CAD build for the part. Positions are in the model's coordinates, mm. A direction names the side the tool comes from. Round coordinates to 2 decimals unless told otherwise and drop trailing zeros. Write each loop counter-clockwise with the first axis right and the second up, starting at its lowest first coordinate (ties: lowest second). Pieces come first, ordered by that corner, then holes. Notation, with made-up numbers: (-38.75, 22.25) - (16.25, 22.25) arc R16 ccw to (16.25, 50.25) - close; hole circle Ø1 at (-24, -31.75). An arc over 180 degrees is marked (long way). Use one line per item in the form item = value. Start each with the question number.
Item 1: Band-saw the part on A-A, the plane y = 50.5. List the corners of the cut face in (x, z).
Item 2: Band-saw the part on B-B, the plane x = 15. Give the number of separate pieces and of enclosed holes in the cut face, and give its area (3 significant figures).
Item 3: Tool access for faces 1 (the flat face through (26.4, 49.1, 6.6)), 2 (the flat face through (15, 65, 0.5)), 3 (the cylindrical face through (23.314, 9.721, 3.254)), 4 (the flat face through (17, 43, 5.7)): list every direction of +Z, -Z, +X, -X, +Y, -Y with a clear straight run to the whole face (end or side of a thin tool).
Item 4: Drill centre lines: L1, parallel to Y at x = 15, z = 3.05 (3 decimals); L2, parallel to Y at x = 25, z = 3; L3, parallel to Y at x = 15, z = 8.35 (3 decimals). Where is each one in solid material? Low to high.
Item 5: Pin check, flat tips, straight feed: pin 1 (3 mm diameter, centred on x = 17, y = 13.5, fed in from -Z); pin 2 (4 mm diameter, centred on x = 5, y = 65.5, fed in from +Z). Stop position of each tip, or through.
Item 6: Pull direction Y, two halves, no side cores. Call faces 5 (the flat face through (15, 0, 5)), 6 (the flat face through (12, 38, 10)), 7 (the flat face through (17, 16, 5.7)): +Y half, -Y half, draft (parallel to the pull), parting line (faces both ways), or undercut.
Autodesk Inventor part; units mm, degrees
ref_plane "YZ Plane" through (0, 0, 0) normal (1, 0, 0) x (0, 1, 0)
ref_plane "XZ Plane" through (0, 0, 0) normal (0, 1, 0) x (-1, 0, 0)
ref_plane "XY Plane" through (0, 0, 0) normal (0, 0, 1) x (1, 0, 0)
sketch "Skizze1" plane through (0, 0, 0) normal (0, 0, 1) x (1, 0, 0)
  line L0 (0, 0) -> (30, 0)
  line L1 (30, 0) -> (30, 75)
  line L2 (30, 75) -> (0, 75)
  line L3 (0, 75) -> (0, 0)
  dimension "d0" = 30
  dimension "d1" = 75
extrude "Extrusion1" add sketch "Skizze1" along normal blind 10
sketch "Skizze2" plane through (0, 0, 10) normal (0, 0, 1) x (1, 0, 0)
  line L0 (5, 65.5) -> (25, 65.5) construction
  line L1 (25, 65.5) -> (25, 50.5) construction
  line L2 (25, 50.5) -> (5, 50.5) construction
  line L3 (5, 50.5) -> (5, 65.5) construction
  line L4 (5, 9.5) -> (25, 9.5) construction
  line L5 (25, 9.5) -> (25, 24.5) construction
  line L6 (25, 24.5) -> (5, 24.5) construction
  line L7 (5, 24.5) -> (5, 9.5) construction
  line L8 (30, 75) -> (0, 75) construction
  line L9 (0, 0) -> (30, 0) construction
  line L10 (15, 65.5) -> (15, 75) construction
  line L11 (15, 50.5) -> (15, 24.5) construction
  dimension "d4" = 9.5
  dimension "d5" = 15
  dimension "d6" = 9.5
  dimension "d7" = 15
  dimension "d8" = 20
hole "Bohrung1" at (5, 65.5, 10) at (25, 65.5, 10) at (25, 50.5, 10) at (5, 50.5, 10) at (5, 24.5, 10) at (25, 24.5, 10) at (25, 9.5, 10) at (5, 9.5, 10) direction (0, 0, -1) diameter 3.4 end through all counterbore diameter 6.5 counterbore depth 3.4
sketch "Skizze4" plane through (0, 0, 0) normal (0, 0, -1) x (-1, 0, 0)
  line L0 (-18.5, 75) -> (-11.5, 75)
  line L1 (-11.5, 75) -> (-11.5, 55)
  line L2 (-11.5, 55) -> (-18.5, 55)
  line L3 (-18.5, 55) -> (-18.5, 75)
  line L4 (-30, 75) -> (0, 75)
  point P0 (0, 0)
  point P1 (-15, 75)
  dimension "d22" = 20
  dimension "d23" = 7
extrude "Extrusion3" cut sketch "Skizze4" against normal blind 0.5
fillet "Rundung1" radius 5 4 edges at (0, 75, 5) (30, 75, 5) (0, 0, 5) (30, 0, 5)
fillet "Rundung3" radius 0.5 4 edges at (18.5, 75, 0.25) (11.5, 75, 0.25) (18.5, 55, 0.25) (11.5, 55, 0.25)
fillet "Rundung2" radius 0.5 24 edges at (1.4645, 73.5355, 10) (0, 37.5, 10) (1.4645, 1.4645, 10) (15, 0, 10) (28.5355, 1.4645, 10) (30, 37.5, 10) (28.5355, 73.5355, 10) (15, 75, 10) (18.6464, 74.8536, 0) (18.5, 65, 0) (18.3536, 55.1464, 0) (15, 55, 0) (11.6464, 55.1464, 0) (11.5, 65, 0) (11.3536, 74.8536, 0) (8, 75, 0) (1.4645, 73.5355, 0) (0, 37.5, 0) (1.4645, 1.4645, 0) (15, 0, 0) (28.5355, 1.4645, 0) (30, 37.5, 0) (28.5355, 73.5355, 0) (22, 75, 0)
sketch "Skizze5" plane through (0, 0, 0) normal (0, 0, -1) x (-1, 0, 0)
  line L0 (-18, 54.5) -> (-12, 54.5) construction
  line L1 (-15, 54.5) -> (-15, 40.875) construction
  line L2 (-15, 40.875) -> (-15, 27.25) construction
  line L3 (-15, 27.25) -> (-15, 13.625) construction
  line L4 (-15, 13.625) -> (-15, 0) construction
  line L5 (-5, 0) -> (-25, 0) construction
  point P0 (0, 0)
hole "Bohrung2" at (15, 13.625, 0) at (15, 27.25, 0) at (15, 40.875, 0) direction (0, 0, 1) diameter 5.5 end through all counterbore diameter 10 counterbore depth 5.7
properties part number "AdapterLinearGuideLong"
Determined:
q1.outline = (0, 0.5) arc R0.5 ccw to (0.5, 0) - (3.3, 0) - (3.3, 6.6) - (1.75, 6.6) - (1.75, 10) - (0.5, 10) arc R0.5 ccw to (0, 9.5) - close; (6.7, 0) - (23.3, 0) - (23.3, 6.6) - (21.75, 6.6) - (21.75, 10) - (8.25, 10) - (8.25, 6.6) - (6.7, 6.6) - close; (26.7, 0) - (29.5, 0) arc R0.5 ccw to (30, 0.5) - (30, 9.5) arc R0.5 ccw to (29.5, 10) - (28.25, 10) - (28.25, 6.6) - (26.7, 6.6) - close
q2.separate_pieces = 4
q2.enclosed_holes = 0
q2.area = 498 mm²
q3.face_1 = +Z
q3.face_2 = -Z, +Y
q3.face_3 = +Z, -Z
q3.face_4 = -Z
q4.L1 = 0 to 8.625, 18.625 to 22.25, 32.25 to 35.875, 45.875 to 75
q4.L2 = 0 to 7.8, 11.2 to 22.8, 26.2 to 48.8, 52.2 to 63.8, 67.2 to 75
q4.L3 = 0 to 10.875, 16.375 to 24.5, 30 to 38.125, 43.625 to 75
q5.pin_1 = 5.7
q5.pin_2 = 6.6
q6.face_5 = -Y half
q6.face_6 = draft
q6.face_7 = undercut
